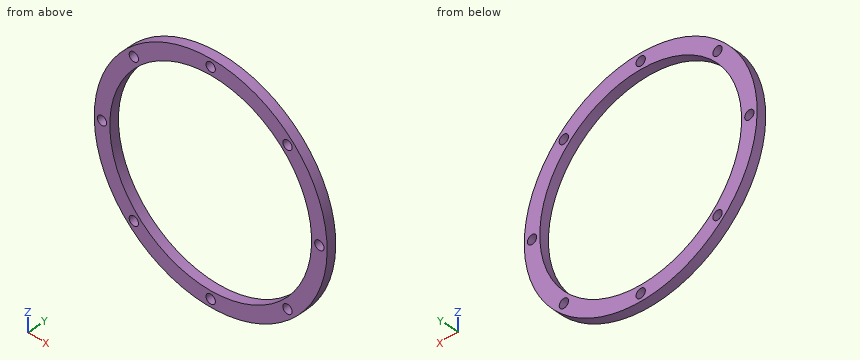
from build123d import *

# Parameters (mm, degrees)
SKETCH_1_R          = 75
EXTRUDE_1_DEPTH     = 6
SKETCH_2_R          = 3
CUT_EXTRUDE_1_DEPTH = 6
SKETCH_3_R          = 65
CUT_EXTRUDE_2_DEPTH = 6


with BuildPart() as part:
    # Эскиз1 → Бобышка-Вытянуть1 (new body)
    with BuildSketch(Plane(origin=(0, 0, 0), x_dir=(1, 0, 0), z_dir=(0, 1, 0))):
        with Locations(Location((0, 0, 0), (0, 0, 270))):
            Circle(SKETCH_1_R)
    extrude(amount=EXTRUDE_1_DEPTH)

    # Эскиз2 → Вырез-Вытянуть1 (cut)
    with BuildSketch(Plane(origin=(0, 6, 0), x_dir=(1, 0, 0), z_dir=(0, 1, 0))):
        with Locations(Location((-70, 0, 0), (0, 0, 270))):
            Circle(SKETCH_2_R)
        with Locations(Location((70, 0, 0), (0, 0, 90))):
            Circle(SKETCH_2_R)
        with Locations(Location((0, -70, 0), (0, 0, 270))):
            Circle(SKETCH_2_R)
        with Locations(Location((0, 70, 0), (0, 0, 90))):
            Circle(SKETCH_2_R)
        with Locations(Location((-49.497474683, -49.497474683, 0), (0, 0, 270))):
            Circle(SKETCH_2_R)
        with Locations(Location((-49.497474683, 49.497474683, 0), (0, 0, 90))):
            Circle(SKETCH_2_R)
        with Locations(Location((49.497474683, -49.497474683, 0), (0, 0, 270))):
            Circle(SKETCH_2_R)
        with Locations(Location((49.497474683, 49.497474683, 0), (0, 0, 90))):
            Circle(SKETCH_2_R)
    extrude(amount=-CUT_EXTRUDE_1_DEPTH, mode=Mode.SUBTRACT)

    # Эскиз3 → Вырез-Вытянуть2 (cut)
    with BuildSketch(Plane(origin=(0, 6, 0), x_dir=(1, 0, 0), z_dir=(0, 1, 0))):
        with Locations(Location((0, 0, 0), (0, 0, 270))):
            Circle(SKETCH_3_R)
    extrude(amount=-CUT_EXTRUDE_2_DEPTH, mode=Mode.SUBTRACT)


solid = part.part
Can you work these out from the model? Positions are in its coordinate system, mm. Give positions to 0.01 mm unless a question says otherwise; leave off trailing zeros. Loops run counter-clockwise (first coordinate to the right, second up) from the corner with the lowest first, then second, coordinate; pieces in that order, holes last. Notation, with made-up numbers: M 69.25,-40 L 123.25,-40 A26 ccw 123.25,-15 Z; hole C 49.25,-9.5 d1. An arc over 180 degrees is marked long. One line per item, written item: value. Start each with the question number.
1) I'm going to push flat-ended pins straight in: pin 1 (5.5 mm diameter, centred on x = -70, z = 0, fed in from -Y); pin 2 (1 mm diameter, centred on x = -39, y = 4.5, fed in from -Z); pin 3 (2 mm diameter, centred on x = 48, y = 5, fed in from +Z). Where does each tip first touch, or does it pass through?
2) If we section it at D-D, the plane z = 43: Write out the boundary of the cut face in (x, y).
3) If I drill on line 1 (X direction, y = 3.3, z = 0); line 2 (Z direction, x = -1, y = 3.85); line 3 (X direction, y = 2.4, z = 56), over which ranges is the centre line in solid material (lowest first)? Write a range as [from, to].
4) If we section it at A-A, the plane x = 70: Write out the boundary of the cut face in (y, z).
5) If we section it at B-B, the plane z = 0: Write out the boundary of the cut face in (x, y), and give its area (3 significant figures).
6) If we section it at C-C, the plane y = 3.2: Give the number of separate pieces and of enclosed holes in the cut face, and give its area (3 significant figures).
Completed:
1. pin 1: passes through
1. pin 2: stops at z = -64.36
1. pin 3: stops at z = 58.45
2. outline: M -61.45,0 L -48.74,0 L -48.74,6 L -61.45,6 Z; M 48.74,0 L 61.45,0 L 61.45,6 L 48.74,6 Z
3. line 1: x = [-75, -73], [-67, -65], [65, 67], [73, 75]
3. line 2: z = [-74.99, -72.83], [-67.17, -64.99], [64.99, 67.17], [72.83, 74.99]
3. line 3: x = [-49.89, -33], [33, 49.89]
4. outline: M 0,-26.93 L 6,-26.93 L 6,-3 L 0,-3 Z; M 0,3 L 6,3 L 6,26.93 L 0,26.93 Z
5. outline: M -75,0 L -73,0 L -73,6 L -75,6 Z; M -67,0 L -65,0 L -65,6 L -67,6 Z; M 65,0 L 67,0 L 67,6 L 65,6 Z; M 73,0 L 75,0 L 75,6 L 73,6 Z
5. area: 48.0 mm^2
6. separate pieces: 1
6. enclosed holes: 9
6. area: 4,170 mm^2
